```python
from build123d import *

# Parameters (mm, degrees)
SALIENTE_EXTRUIR1_DEPTH = 14
CROQUIS2_R              = 4.25
CORTAR_EXTRUIR1_DEPTH   = 15


with BuildPart() as part:
    # Croquis1 → Saliente-Extruir1 (new body)
    with BuildSketch(Plane(origin=(0, 0, 0), x_dir=(1, 0, 0), z_dir=(0, 1, 0))):
        Polygon((150, -240), (210, -240), (210, 240), (-210, 240), (-210, -240), (-150, -240), (-150, -160), (150, -160), align=None)
    extrude(amount=SALIENTE_EXTRUIR1_DEPTH)

    # Croquis2 → Cortar-Extruir1 (cut, through all)
    with BuildSketch(Plane(origin=(0, 14, 0), x_dir=(1, 0, 0), z_dir=(0, 1, 0))):
        with Locations((-182.5, -230.00000008)):
            Circle(CROQUIS2_R)
        with Locations((-182.5, -170.00000008)):
            Circle(CROQUIS2_R)
        with Locations((-192.5, -58)):
            Circle(CROQUIS2_R)
        with Locations((-192.5, 199.388515843)):
            Circle(CROQUIS2_R)
        with Locations((192.499514399, 200)):
            Circle(CROQUIS2_R)
        with Locations((192.5, -58)):
            Circle(CROQUIS2_R)
        with Locations((182.5, -170)):
            Circle(CROQUIS2_R)
        with Locations((182.5, -230)):
            Circle(CROQUIS2_R)
    extrude(amount=-CORTAR_EXTRUIR1_DEPTH, mode=Mode.SUBTRACT)


solid = part.part
```
Geometry: final body of the model. Coordinates: model frame, mm. A direction names the side the tool comes from. Coordinates: 2 decimals unless noted, no trailing zeros. Loops run counter-clockwise (first coordinate to the right, second up) from the corner with the lowest first, then second, coordinate; pieces in that order, holes last. Notation, with made-up numbers: (22.5, 5.5) -> (75.5, 5.5) arc R21 cw to (75.5, 36.5) -> close; hole circle Ø7 at (36, -8.75). An arc over 180 degrees is marked (long way). Use a Markdown table: item, result. Add a question column.
(1) Line query: line 1 along Z through (x, y) = (-192.5, 11.25); line 2 along X through (y, z) = (5.75, -200); line 3 along X through (y, z) = (5, 58). Output: solid intervals per line, ascending.
(2) Pin query (flat end, axial travel): pin 1 Ø7.5 at (x, z) = (-192.5, 58) entering from -Y; pin 2 Ø7 at (x, y) = (35, 8.5) entering from +Z. Return the tip coordinate at first contact, or that it passes through.
(3) Section query B-B, the plane y = 10.75. State how many separate pieces and enclosed holes the cut face has, plus the area to 3 significant figures.
(4) Access query for faces 1 (the flat face through (-2, 7, 160)), 2 (the flat face through (210, 7, 3)). Directions: +Z, -Z, +X, -X, +Y, -Y. A direction counts if a zero-diameter tool reaches every point of the face in a straight line with its end or side. Return the directions, or none.
(5) Section query A-A, the plane x = -123.5. Return loops of the section in (y, z), plus the area to 3 significant figures.
Answer:
| question | item | result |
|---|---|---|
| 1 | line 1 | z = -240 to -203.64, -195.14 to 53.75, 62.25 to 240 |
| 1 | line 2 | x = -210 to -196.71, -188.29 to 188.25, 196.75 to 210 |
| 1 | line 3 | x = -210 to -196.75, -188.25 to 188.25, 196.75 to 210 |
| 2 | pin 1 | passes through |
| 2 | pin 2 | stops at z = 160 |
| 3 | separate pieces | 1 |
| 3 | enclosed holes | 8 |
| 3 | area | 177,000 mm^2 |
| 4 | face 1 | +Z, +Y, -Y |
| 4 | face 2 | +Z, -Z, +X, +Y, -Y |
| 5 | outline | (0, -240) -> (14, -240) -> (14, 160) -> (0, 160) -> close |
| 5 | area | 5,600 mm^2 |
